```python
from build123d import *

# Parameters (mm, degrees)
SKETCH1_W            = 210
SKETCH1_H            = 80
SKETCH1_R            = 11.9875
BOSS_EXTRUDE1_DEPTH  = 6.35
M5_CLEARANCE_HOLE1_D = 5.3
FILLET1_R            = 5
M8_CLEARANCE_HOLE2_D = 8.4


with BuildPart() as part:
    # Sketch1 → Boss-Extrude1 (new body)
    with BuildSketch(Plane.XY):
        with Locations((35, 0)):
            Rectangle(SKETCH1_W, SKETCH1_H)
        Circle(SKETCH1_R, mode=Mode.SUBTRACT)
    extrude(amount=-BOSS_EXTRUDE1_DEPTH)

    # M5 Clearance Hole1 (through all)
    with Locations(Plane(origin=(-30, 30, 0), x_dir=(1, 0, 0), z_dir=(0, 0, 1))):
        with Locations((0, 0), (0, -60), (130, -60), (130, 0)):
            Hole(M5_CLEARANCE_HOLE1_D / 2)

    # Fillet1
    fillet1_edges = [part.edges().sort_by_distance(p)[0] for p in [
        (-70, 40, -3.175),
        (140, 40, -3.175),
        (140, -40, -3.175),
        (-70, -40, -3.175),
    ]]
    fillet(fillet1_edges, radius=FILLET1_R)

    # M8 Clearance Hole2 (through all)
    with Locations(Plane(origin=(-50, 12.5, 0), x_dir=(1, 0, 0), z_dir=(0, 0, 1))):
        with Locations((0, 0), (0, -25), (170, -25), (170, 0)):
            Hole(M8_CLEARANCE_HOLE2_D / 2)


solid = part.part
```
CAD build for the part. Positions are in the model's coordinates, mm. Coordinates: 2 decimals unless noted, no trailing zeros. Loops run counter-clockwise (first coordinate to the right, second up) from the corner with the lowest first, then second, coordinate; pieces in that order, holes last. Notation, with made-up numbers: (10, -22) - (33, -22) arc R16 cw to (33, -1) - close; hole circle Ø1 at (-30, -8.5). An arc over 180 degrees is marked (long way). Use CSV: the item, a comma, the result in double quotes. Start each with the question number.
Q1. Two-plate mould, pull along X, no slides. Class faces 1 (the flat face through (34, 1, 0)), 2 (the cylindrical face through (100.34, -27.37, -3.22)), 3 (the cylindrical face through (116.12, -14.11, -3.22)), 4 (the cylindrical face through (138, -39, -3)): +X half, -X half, draft (parallel to the pull), parting line (faces both ways), or undercut.
Q2. Cut at A-A, the plane x = 100. List the corners of the cut face in (y, z).
Q3. Probe probe 1 along Y at (x, z) = (100, -4.5); probe 2 along Y at (x, z) = (0, -1.5); probe 3 along Y at (x, z) = (-50, -1.25). List the from-to ranges inside material, lowest first. Write a range as from..to.
Q4. Cut at C-C, the plane y = -30. List the corners of the cut face in (x, z).
Q5. Drop a flat-ended pin along its axis: P1, Ø3, axis at x = -30, y = -30, coming from the +Z side. Give the stop position or say it passes through.
Q6. Cut at D-D, the plane z = -5.25. State how many separate pieces and enclosed holes the cut face has, then the cut area to 3 significant figures.
Q7. Cut at B-B, the plane y = 0. List the corners of the cut face in (x, z), then the cut area to 3 significant figures.
Here are the results:
1,face 1,"draft"
1,face 2,"undercut"
1,face 3,"undercut"
1,face 4,"+X half"
2,outline,"(-40, -6.35) - (-32.65, -6.35) - (-32.65, 0) - (-40, 0) - close; (-27.35, -6.35) - (27.35, -6.35) - (27.35, 0) - (-27.35, 0) - close; (32.65, -6.35) - (40, -6.35) - (40, 0) - (32.65, 0) - close"
3,probe 1,"-40..-32.65, -27.35..27.35, 32.65..40"
3,probe 2,"-40..-11.99, 11.99..40"
3,probe 3,"-40..-16.7, -8.3..8.3, 16.7..40"
4,outline,"(-70, -6.35) - (-32.65, -6.35) - (-32.65, 0) - (-70, 0) - close; (-27.35, -6.35) - (97.35, -6.35) - (97.35, 0) - (-27.35, 0) - close; (102.65, -6.35) - (140, -6.35) - (140, 0) - (102.65, 0) - close"
5,P1,"through"
6,separate pieces,"1"
6,enclosed holes,"9"
6,area,"16,000 mm2"
7,outline,"(-70, -6.35) - (-11.99, -6.35) - (-11.99, 0) - (-70, 0) - close; (11.99, -6.35) - (140, -6.35) - (140, 0) - (11.99, 0) - close"
7,area,"1,180 mm2"
